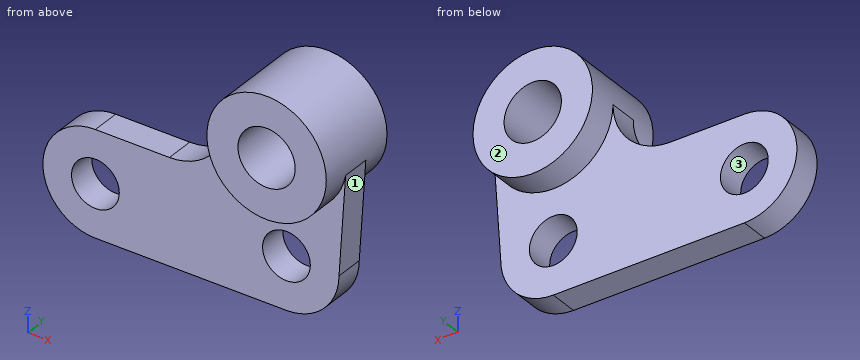
```python
from build123d import *

# Parameters (mm, degrees)
F0_R     = 10
F1_DEPTH = 6
F2_R     = 25
F2_R_2   = 12
F3_DEPTH = 18
F4_R     = 23.9999


# Not quite as in the source:
# - a fillet or chamfer is up to 0.001 mm smaller than in the source, because OpenCascade refuses the exact size


with BuildPart() as f1:
    # F0 (on Front) → F1 (new body, symmetric)
    with BuildSketch(Plane.XZ):
        with BuildLine():
            Line((16.57635398, 22), (-38.42364602, 22))
            ThreePointArc((-38.42364602, 22), (-60.42364602, 0), (-38.42364602, -22))
            Line((-38.42364602, -22), (41.57635398, -22))
            ThreePointArc((41.57635398, -22), (57.1327031661, -15.5563491861), (63.57635398, 0))
            Line((63.57635398, 0), (66.521399326, 44.3432825568))
            ThreePointArc((66.521399326, 44.3432825568), (40.7475396611, 21.0137424406), (16.57635398, 46))
            Line((16.57635398, 46), (16.57635398, 22))
        make_face()
        with Locations((-38.42364602, 0)):
            Circle(F0_R, mode=Mode.SUBTRACT)
        with Locations((41.57635398, 0)):
            Circle(F0_R, mode=Mode.SUBTRACT)
    extrude(amount=F1_DEPTH, both=True)

    # F2 (on Front) → F3 (join, symmetric)
    with BuildSketch(Plane.XZ):
        with Locations((41.726754687, 46.0397801568)):
            Circle(F2_R)
        with Locations((41.726754687, 46.0397801568)):
            Circle(F2_R_2, mode=Mode.SUBTRACT)
    extrude(amount=F3_DEPTH, both=True)

    # F4 (radius 24 in the source; OpenCascade refuses exactly that, so slightly less here)
    f4_edges = [f1.edges().sort_by_distance(p)[0] for p in [
        (16.576354, 0, 22),
    ]]
    fillet(f4_edges, radius=F4_R)


solid = f1.part
```
Work out the finished part from the listing and answer in its coordinate system (mm). Face numbers are marked on the shaded views. Coordinates: 2 decimals unless noted, no trailing zeros. Loops run counter-clockwise (first coordinate to the right, second up) from the corner with the lowest first, then second, coordinate; pieces in that order, holes last. Notation, with made-up numbers: (52.5, 16) -> (96.5, 16) arc R30 cw to (96.5, 50) -> close; hole circle Ø11 at (-13, -34.75). An arc over 180 degrees is marked (long way). Answer as CSV lines item,"result".
Q1. The part is cut by section C-C on y = -4. Write down the section's boundary in (x, z), and give its area (3 significant figures).
Findings:
outline,"(-38.42, -22) -> (41.58, -22) arc R22 ccw to (63.58, 0) -> (66.35, 41.69) arc R25 ccw (long way) to (48.04, 21.85) arc R25 cw to (16.58, 46) arc R24 cw to (-7.42, 22) -> (-38.42, 22) arc R22 ccw to start; hole circle Ø20 at (-38.42, 0); hole circle Ø24 at (41.73, 46.04); hole circle Ø20 at (41.58, 0)"
area,"6,360 mm²"
Q2. The part is cut by section B-B on x = 25. Write down the section's boundary in (y, z).
Findings:
outline,"(-18, 27.46) -> (18, 27.46) -> (18, 64.62) -> (-18, 64.62) -> close; (-6, -22) -> (6, -22) -> (6, 27.29) -> (-6, 27.29) -> close"
Q3. Each of these flat-tipped pins is pushed along its axis until it touches: pin 1 (23 mm diameter, centred on x = 41.58, z = 0, fed in from +Y); pin 2 (4 mm diameter, centred on y = -0.5, z = 54, fed in from +X); pin 3 (3.5 mm diameter, centred on x = -16, y = 1.5, fed in from +Z); pin 4 (1.5 mm diameter, centred on x = 10.5, z = 32.5, fed in from -Y). Where does it stop, or does it pass through?
Findings:
pin 1,"stops at y = 6"
pin 2,"stops at x = 66.01"
pin 3,"stops at z = 22"
pin 4,"passes through"
Q4. The part is cut by section A-A on z = 5. Write down the section's boundary in (x, y), and give its area (3 significant figures).
Findings:
outline,"(-59.85, -6) -> (-47.08, -6) -> (-47.08, 6) -> (-59.85, 6) -> close; (-29.76, -6) -> (32.92, -6) -> (32.92, 6) -> (-29.76, 6) -> close; (50.24, -6) -> (63.91, -6) -> (63.91, 6) -> (50.24, 6) -> close"
area,"1,070 mm²"
Q5. For a pull along X with two mould halves and no side action, classify the marked faces 1, 2 and 3 as +X half, -X half, draft (parallel to the pull), parting line (faces both ways), or undercut.
Findings:
face 1,"+X half"
face 2,"draft"
face 3,"undercut"
Q6. The part is cut by section D-D on x = 44.5. Write down the section's boundary in (y, z).
Findings:
outline,"(-18, 21.19) -> (18, 21.19) -> (18, 34.36) -> (-18, 34.36) -> close; (-18, 57.71) -> (18, 57.71) -> (18, 70.89) -> (-18, 70.89) -> close; (-6, -21.8) -> (6, -21.8) -> (6, -9.56) -> (-6, -9.56) -> close; (-6, 9.56) -> (6, 9.56) -> (6, 21.17) -> (-6, 21.17) -> close"
Q7. Find the intervals of material crossed by probe 1 along X at (y, z) = (-15.5, 46.5); probe 2 along X at (y, z) = (1.5, -5.5); probe 3 along Y at (x, z) = (-16, -3.5), in increasing order.
Findings:
probe 1,"x = 16.73 to 29.74, 53.72 to 66.72"
probe 2,"x = -59.73 to -46.78, -30.07 to 33.22, 49.93 to 62.88"
probe 3,"y = -6 to 6"
